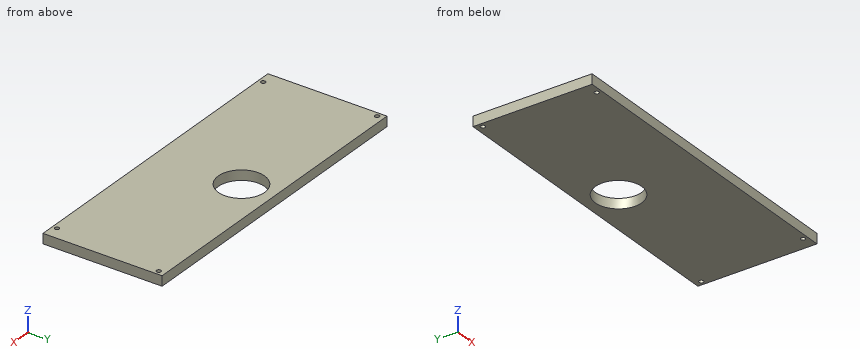
from build123d import *

# Parameters (mm, degrees)
SKETCH1_W           = 304.8
SKETCH1_H           = 114.3
SKETCH1_R           = 22.225
BOSS_EXTRUDE1_DEPTH = 9.525
SKETCH2_R           = 2.159
CUT_EXTRUDE1_DEPTH  = 10.525


with BuildPart() as part:
    # Sketch1 → Boss-Extrude1 (new body)
    with BuildSketch(Plane.XY):
        with Locations((0, -25.4)):
            Rectangle(SKETCH1_W, SKETCH1_H)
        Circle(SKETCH1_R, mode=Mode.SUBTRACT)
    extrude(amount=BOSS_EXTRUDE1_DEPTH)

    # Sketch2 → Cut-Extrude1 (cut, through all)
    with BuildSketch(Plane.XY.offset(9.525)):
        with Locations((-139.7, -78.105)):
            Circle(SKETCH2_R)
        with Locations((-147.955, 25.4)):
            Circle(SKETCH2_R)
        with Locations((147.955, 25.4)):
            Circle(SKETCH2_R)
        with Locations((139.7, -78.105)):
            Circle(SKETCH2_R)
    extrude(amount=-CUT_EXTRUDE1_DEPTH, mode=Mode.SUBTRACT)


solid = part.part
The listing builds one solid part. Answer for the finished solid, in the listing's coordinates (mm). Round coordinates to 2 decimals unless told otherwise and drop trailing zeros. Order: outer loops, then holes, each group sorted by start corner. A loop starts at its lowest first (then second) coordinate and runs counter-clockwise, first axis right, second up. Notation, with made-up numbers: (21, 41.5) -> (55, 41.5) arc R16 ccw to (55, 53.5) -> close; hole circle Ø6 at (4.25, 44). An arc over 180 degrees is marked (long way). Write each question's results on one line, items separated by ' | '. Start each with the question number.
Q1. Find section B-B (y = 0). Determine the outline of the cut face in (x, z) (3 decimals).
Q2. Find section C-C (z = 1.5). Determine the outline of the cut face in (x, y) (3 decimals).
Q3. Straight lines are drawn through the part: probe 1 along Y at (x, z) = (-139.7, 7.25); probe 2 along Y at (x, z) = (0, 5) (3 decimals); probe 3 along X at (y, z) = (27, 4). For each, find the intervals that lie inside material, in ascending order. Write a range as from..to.
Q4. Find section A-A (x = 0). Determine the outline of the cut face in (y, z) (3 decimals).
Worked answers:
1) outline: (-152.4, 0) -> (-22.225, 0) -> (-22.225, 9.525) -> (-152.4, 9.525) -> close; (22.225, 0) -> (152.4, 0) -> (152.4, 9.525) -> (22.225, 9.525) -> close
2) outline: (-152.4, -82.55) -> (152.4, -82.55) -> (152.4, 31.75) -> (-152.4, 31.75) -> close; hole circle Ø4.318 at (-147.955, 25.4); hole circle Ø4.318 at (-139.7, -78.105); hole circle Ø44.45 at (0, 0); hole circle Ø4.318 at (139.7, -78.105); hole circle Ø4.318 at (147.955, 25.4)
3) probe 1: y = -82.55..-80.26, -75.95..31.75 | probe 2: y = -82.55..-22.225, 22.225..31.75 | probe 3: x = -152.4..-149.4, -146.51..146.51, 149.4..152.4
4) outline: (-82.55, 0) -> (-22.225, 0) -> (-22.225, 9.525) -> (-82.55, 9.525) -> close; (22.225, 0) -> (31.75, 0) -> (31.75, 9.525) -> (22.225, 9.525) -> close
